Geometry: final body of the model. Coordinates: model frame, mm. Round coordinates to 2 decimals unless told otherwise and drop trailing zeros. Write each loop counter-clockwise with the first axis right and the second up, starting at its lowest first coordinate (ties: lowest second). Pieces come first, ordered by that corner, then holes. Notation, with made-up numbers: (42.5, 1) - (71.5, 1) arc R20 cw to (71.5, 24) - close; hole circle Ø1 at (-32, -14.5). An arc over 180 degrees is marked (long way). Write each question's results on one line, items separated by ' | '.
from build123d import *

# Parameters (mm, degrees)
BOSS_EXTRUDE1_DEPTH = 7
CUT_EXTRUDE1_DEPTH  = 5


with BuildPart() as part:
    # Sketch2 → Boss-Extrude1 (new body)
    with BuildSketch(Plane(origin=(0, 0, 0), x_dir=(1, 0, 0), z_dir=(0, 1, 0))):
        with BuildLine():
            Line((10, 0), (272, 0))
            ThreePointArc((272, 0), (279.071067812, 2.928932188), (282, 10))
            Line((282, 10), (282, 175.95))
            ThreePointArc((282, 175.95), (279.071067812, 183.021067812), (272, 185.95))
            Line((272, 185.95), (10, 185.95))
            ThreePointArc((10, 185.95), (2.928932188, 183.021067812), (0, 175.95))
            Line((0, 175.95), (0, 10))
            ThreePointArc((0, 10), (2.928932188, 2.928932188), (10, 0))
        make_face()
    extrude(amount=BOSS_EXTRUDE1_DEPTH)

    # Sketch3 → Cut-Extrude1 (cut)
    with BuildSketch(Plane(origin=(0, 7, 0), x_dir=(1, 0, 0), z_dir=(0, 1, 0))):
        Polygon((74, 16), (90, 16), (90, 42), (74, 42), (74, 51.5), (90, 51.5), (90, 80), (74, 80), (74, 84), (12, 84), (12, 12), (74, 12), align=None)
        Polygon((180, 42), (164, 42), (164, 51.5), (180, 51.5), (180, 80), (164, 80), (164, 84), (102, 84), (102, 12), (164, 12), (164, 16), (180, 16), align=None)
        Polygon((270, 42), (254, 42), (254, 51.5), (270, 51.5), (270, 80), (254, 80), (254, 84), (192, 84), (192, 12), (254, 12), (254, 16), (270, 16), align=None)
        Polygon((180, 132), (164, 132), (164, 141.5), (180, 141.5), (180, 170), (164, 170), (164, 174), (102, 174), (102, 102), (164, 102), (164, 106), (180, 106), align=None)
        Polygon((270, 132), (254, 132), (254, 141.5), (270, 141.5), (270, 170), (254, 170), (254, 174), (192, 174), (192, 102), (254, 102), (254, 106), (270, 106), align=None)
        Polygon((90, 132), (74, 132), (74, 141.5), (90, 141.5), (90, 170), (74, 170), (74, 174), (12, 174), (12, 102), (74, 102), (74, 106), (90, 106), align=None)
    extrude(amount=-CUT_EXTRUDE1_DEPTH, mode=Mode.SUBTRACT)


solid = part.part
Q1. Pin query (flat end, axial travel): pin 1 (3 mm diameter, centred on x = 33.5, z = -72, fed in from +Y). Return the tip coordinate at first contact, or that it passes through.
Answer block:
pin 1: y = 2
Q2. Section query B-B, the plane x = 69. Return loops of the section in (y, z), plus the area to 3 significant figures.
Answer block:
outline: (0, -185.95) - (7, -185.95) - (7, -174) - (2, -174) - (2, -102) - (7, -102) - (7, -84) - (2, -84) - (2, -12) - (7, -12) - (7, 0) - (0, 0) - close | area: 582 mm2
Q3. Mould query, pull axis Z, two halves, no side actions, for faces 1 (the flat face through (230, 2, -49)), 2 (the cylindrical face through (279.15, 3.45, -182.94)), 3 (the flat face through (139, 0, -94)). Classes: pulls with the +Z half, pulls with the -Z half, needs draft (parallel to the pull), parting line crosses it, or undercut.
Answer block:
face 1: undercut | face 2: pulls with the -Z half | face 3: needs draft
Q4. Section query A-A, the plane z = -128. Return loops of the section in (x, y), plus the area to 3 significant figures.
Answer block:
outline: (0, 0) - (282, 0) - (282, 7) - (270, 7) - (270, 2) - (192, 2) - (192, 7) - (180, 7) - (180, 2) - (102, 2) - (102, 7) - (90, 7) - (90, 2) - (12, 2) - (12, 7) - (0, 7) - close | area: 804 mm2
Q5. Ray query, line 1 along Z through (x, y) = (257, 3.5); line 2 along X through (y, z) = (5.25, -18.5); line 3 along X through (y, z) = (5.25, -173.5). Return the intervals inside material, ascending.
Answer block:
line 1: -185.95 to -170, -141.5 to -132, -106 to -80, -51.5 to -42, -16 to 0 | line 2: 0 to 12, 90 to 102, 180 to 192, 270 to 282 | line 3: 0 to 12, 74 to 102, 164 to 192, 254 to 282
Q6. Section query C-C, the plane y = 4. Give the number of separate pieces and of enclosed holes in the cut face, plus the area to 3 significant figures.
Answer block:
separate pieces: 1 | enclosed holes: 6 | area: 20,300 mm2
